The listing builds one solid part. Answer for the finished solid, in the listing's coordinates (mm). Face numbers are marked on the shaded views. Coordinates: 2 decimals unless noted, no trailing zeros. Loops run counter-clockwise (first coordinate to the right, second up) from the corner with the lowest first, then second, coordinate; pieces in that order, holes last. Notation, with made-up numbers: (-30.75, 46.25) -> (-12.75, 46.25) arc R24 ccw to (-12.75, 76.25) -> close; hole circle Ø1 at (58, 45.5). An arc over 180 degrees is marked (long way). Answer in a Markdown table with one row per item.
```python
from build123d import *

# Parameters (mm, degrees)
SKETCH1_R           = 2.3
BOSS_EXTRUDE1_DEPTH = 12.9
BOSS_EXTRUDE2_START = 6.45
SKETCH2_R           = 4
SKETCH2_R_2         = 2.3
BOSS_EXTRUDE2_DEPTH = 1
BOSS_EXTRUDE3_START = -6.45
SKETCH2_3_R         = 4
SKETCH2_3_R_2       = 2.3
BOSS_EXTRUDE3_DEPTH = 1


with BuildPart() as part:
    # Sketch1 → Boss-Extrude1 (new body)
    with BuildSketch(Plane(origin=(0, 0, 0), x_dir=(1, 0, 0), z_dir=(0, 1, 0))):
        Circle(SKETCH1_R)
    extrude(amount=BOSS_EXTRUDE1_DEPTH)

    # Sketch2 → Boss-Extrude2 (add)
    with BuildSketch(Plane(origin=(0, 6.45, 0), x_dir=(1, 0, 0), z_dir=(0, 1, 0)).offset(BOSS_EXTRUDE2_START)):
        Circle(SKETCH2_R)
        Circle(SKETCH2_R_2, mode=Mode.SUBTRACT)
    extrude(amount=-BOSS_EXTRUDE2_DEPTH)

    # Sketch2<3> → Boss-Extrude3 (add)
    with BuildSketch(Plane(origin=(0, 6.45, 0), x_dir=(1, 0, 0), z_dir=(0, 1, 0)).offset(BOSS_EXTRUDE3_START)):
        Circle(SKETCH2_3_R)
        Circle(SKETCH2_3_R_2, mode=Mode.SUBTRACT)
    extrude(amount=BOSS_EXTRUDE3_DEPTH)


solid = part.part
```
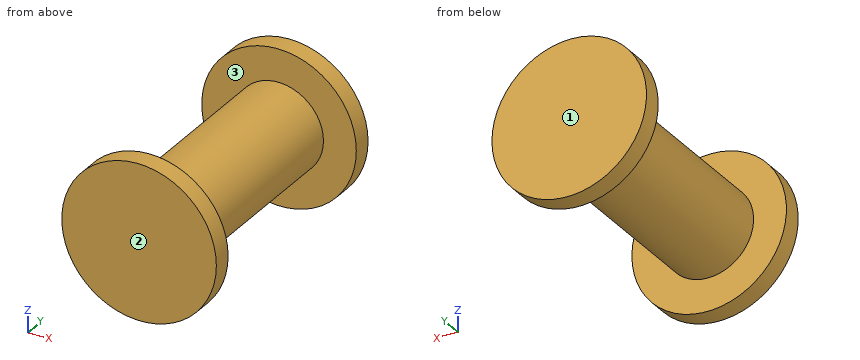
Item 1: Flat-ended cylindrical pins translate along their axes: pin 1 Ø2 at (x, y) = (1, 9) entering from +Z; pin 2 Ø1 at (x, y) = (-1, 5.5) entering from +Z (3 decimals); pin 3 Ø2 at (x, y) = (-2.5, 7.5) entering from -Z. Find the tip coordinate at first contact, or state that the pin passes through.
Findings below:
| item | result |
|---|---|
| pin 1 | stops at z = 2.3 |
| pin 2 | stops at z = 2.245 |
| pin 3 | stops at z = -1.74 |
Item 2: Determine the mould class of the marked faces 1, 2 and 3 for opening direction Y: +Y half, -Y half, draft (parallel to the pull), parting line (faces both ways), or undercut.
Findings below:
| item | result |
|---|---|
| face 1 | +Y half |
| face 2 | -Y half |
| face 3 | undercut |
Item 3: A cutting plane is placed at A-A, the plane x = 3.5. Determine the outline of the cut face in (y, z).
Findings below:
| item | result |
|---|---|
| outline | (0, -1.94) -> (1, -1.94) -> (1, 1.94) -> (0, 1.94) -> close; (11.9, -1.94) -> (12.9, -1.94) -> (12.9, 1.94) -> (11.9, 1.94) -> close |
Item 4: A cutting plane is placed at B-B, the plane z = -2.5. Determine the outline of the cut face in (x, y).
Findings below:
| item | result |
|---|---|
| outline | (-3.12, 0) -> (3.12, 0) -> (3.12, 1) -> (-3.12, 1) -> close; (-3.12, 11.9) -> (3.12, 11.9) -> (3.12, 12.9) -> (-3.12, 12.9) -> close |
Item 5: Find the intervals of material crossed by probe 1 along Y at (x, z) = (-2.5, 2); probe 2 along X at (y, z) = (3.25, 1.5); probe 3 along Z at (x, y) = (-0.5, 1.75) (3 decimals), in increasing order.
Findings below:
| item | result |
|---|---|
| probe 1 | y = 0 to 1, 11.9 to 12.9 |
| probe 2 | x = -1.74 to 1.74 |
| probe 3 | z = -2.245 to 2.245 |
Item 6: A cutting plane is placed at C-C, the plane z = 0. Determine the outline of the cut face in (x, y), plus the area to 3 significant figures.
Findings below:
| item | result |
|---|---|
| outline | (-4, 0) -> (4, 0) -> (4, 1) -> (2.3, 1) -> (2.3, 11.9) -> (4, 11.9) -> (4, 12.9) -> (-4, 12.9) -> (-4, 11.9) -> (-2.3, 11.9) -> (-2.3, 1) -> (-4, 1) -> close |
| area | 66.1 mm2 |
Item 7: A cutting plane is placed at D-D, the plane x = 0. Determine the outline of the cut face in (y, z).
Findings below:
| item | result |
|---|---|
| outline | (0, -4) -> (1, -4) -> (1, -2.3) -> (11.9, -2.3) -> (11.9, -4) -> (12.9, -4) -> (12.9, 4) -> (11.9, 4) -> (11.9, 2.3) -> (1, 2.3) -> (1, 4) -> (0, 4) -> close |
